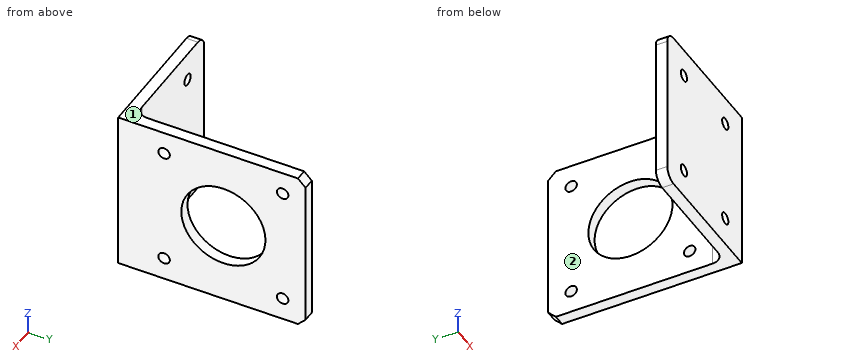
Autodesk Inventor part; units mm, degrees
ref_plane "YZ Plane" through (0, 0, 0) normal (1, 0, 0) x (0, 1, 0)
ref_plane "XZ Plane" through (0, 0, 0) normal (0, 1, 0) x (-1, 0, 0)
ref_plane "XY Plane" through (0, 0, 0) normal (0, 0, 1) x (1, 0, 0)
sketch "Szkic1" plane through (0, 0, 0) normal (0, 0, 1) x (1, 0, 0)
  line L0 (-15.1556, -3.6171) -> (-15.1556, -6.6171)
  line L1 (-15.1556, -6.6171) -> (20.8444, -6.6171)
  line L2 (20.8444, -6.6171) -> (20.8444, 42.3829)
  line L3 (20.8444, 42.3829) -> (17.8444, 42.3829)
  line L4 (17.8444, 42.3829) -> (17.8444, -3.6171)
  line L5 (17.8444, -3.6171) -> (-15.1556, -3.6171)
  point P0 (0, 0)
  dimension "d0" = 3
  dimension "d1" = 36
  dimension "d2" = 49
  dimension "d3" = 3
extrude "Wyciągnięcie proste1" add sketch "Szkic1" along normal blind 43
fillet "Zaokrąglenie1" radius 3 1 edges at (17.8444, -3.6171, 21.5)
sketch "Szkic2" plane through (17.8444, 42.3829, 0) normal (-1, 0, 0) x (0, 0, 1)
  circle A0 centre (21.5033, -21.5) radius 11
  circle A1 centre (21.5, -21.5) radius 16.25
  line L0 (0, 0) -> (0, -43)
  line L1 (0, 0) -> (43, 0)
  line L2 (43, 0) -> (43, -43)
  line L3 (0.5, -0.5) -> (42.5, -0.5)
  line L4 (42.5, -0.5) -> (42.5, -42.5)
  line L5 (42.5, -42.5) -> (0.5, -42.5)
  line L6 (0.5, -42.5) -> (0.5, -0.5)
  point P0 (0, -42.3829)
  point P1 (37, -37)
  point P2 (37, -6)
  point P3 (6, -6)
  point P4 (6, -37)
  dimension "d61" = 42
  dimension "d62" = 42
  dimension "d63" = 0.5
  dimension "d64" = 0.5
  dimension "d65" = 5.5
  dimension "d66" = 5.5
  dimension "d67" = 5.5
  dimension "d68" = 5.5
  dimension "d69" = 5.5
  dimension "d70" = 5.5
  dimension "d71" = 5.5
  dimension "d72" = 5.5
  dimension "d73" = 21
  dimension "d74" = 21
extrude "Wyciągnięcie proste2" cut sketch "Szkic2" against normal blind 43 contours A0
hole "Otwór1" at (17.8444, 5.3829, 6) at (17.8444, 36.3829, 6) at (17.8444, 36.3829, 37) at (17.8444, 5.3829, 37) direction (1, 0, 0) diameter 3 end through all
chamfer "Faza1" distance 2 angle 45 2 edges at (19.3444, 42.3829, 43) (19.3444, 42.3829, 0)
fillet "Zaokrąglenie2" radius 3 2 edges at (-15.1556, -5.1171, 0) (-15.1556, -5.1171, 43)
sketch "Szkic3" plane through (20.8444, -6.6171, 0) normal (0, -1, 0) x (1, 0, 0)
  arc A0 (-33, 43) -> (-36, 40) centre (-33, 40) ccw
  line L0 (-36, 3) -> (-36, 40)
  arc A1 (-36, 3) -> (-33, 0) centre (-33, 3) ccw
  line L1 (-33, 0) -> (0, 0)
  line L2 (0, 0) -> (0, 43)
  line L3 (-33, 43) -> (0, 43)
  point P0 (-20.8444, 0)
  point P1 (-28, 7.5)
  point P2 (-8, 7.5)
  point P3 (-28, 35.5)
  point P4 (-8, 35.5)
  dimension "d32" = 20
  dimension "d33" = 20
  dimension "d34" = 36
  dimension "d35" = 8
  dimension "d36" = 8
  dimension "d37" = 7.5
  dimension "d38" = 7.5
  dimension "d39" = 7.5
  dimension "d40" = 7.5
hole "Otwór2" at (-7.1556, -6.6171, 7.5) at (12.8444, -6.6171, 7.5) at (-7.1556, -6.6171, 35.5) at (12.8444, -6.6171, 35.5) direction (0, 1, 0) diameter 3 end through all
sketch "Szkic4" plane through (14.8444, -3.6171, 43) normal (0, 1, 0) x (1, 0, 0)
  circle A0 centre (-2, 7.5) radius 1.5
  circle A1 centre (-2, 35.5) radius 1.5
  circle A2 centre (-2, 7.5) radius 3.1
  circle A3 centre (-2, 35.5) radius 3.1
  point P0 (-14.8444, 43)
  dimension "d48" = 6.2
  dimension "d49" = 6.2
extrude "Wyciągnięcie proste3" cut sketch "Szkic4" along normal blind 2
properties part number "CNCM_ALU_X_Axis_Nema_17_Mount"
For this review, take the finished solid that the model builds, in its own axes (mm). Face numbers are marked on the shaded views. A direction names the side the tool comes from. Give positions to 0.01 mm unless a question says otherwise; leave off trailing zeros. Order: outer loops, then holes, each group sorted by start corner. A loop starts at its lowest first (then second) coordinate and runs counter-clockwise, first axis right, second up. Notation, with made-up numbers: (65, 70.25) - (107, 70.25) arc R23 ccw to (107, 80.25) - close; hole circle Ø7 at (14, 44.25). An arc over 180 degrees is marked (long way). Answer as a JSON object with one key per item and string values. Group by question number.
Item 1: Take a section at C-C on y = 4.5. Give the boundary of the cut face in (x, z).
Item 2: Take a section at B-B on z = 22. Give the boundary of the cut face in (x, y), and give its area (3 significant figures).
Item 3: Clearance check with flat-ended pins moving along their axes: pin 1 Ø4 at (y, z) = (36.38, 6) entering from -X; pin 2 Ø2.5 at (y, z) = (36.38, 37) entering from -X; pin 3 Ø1.5 at (x, z) = (12.5, 10.5) entering from +Y. State where each tip first meets the part, or that it passes through.
Item 4: Take a section at A-A on y = 19. Give the boundary of the cut face in (x, z).
Item 5: Machinability: for the marked faces 1 and 2, which of the approach directions +Z, -Z, +X, -X, +Y, -Y give a long, thin tool a straight path to every point of the face, cutting with its end or side? Answer none if there is none.
Item 6: Wall thickness on line 1 along Y through (x, z) = (18.85, 37); line 2 along X through (y, z) = (-4, 35); line 3 along X through (y, z) = (4, 10): over which ranges is each line inside the solid? List them lowest first.
Item 7: Take a section at D-D on x = -1.5. Give the boundary of the cut face in (y, z).
Reported:
{
 "1": {"outline": "(17.84, 0) - (20.84, 0) - (20.84, 4.79) - (17.84, 4.79) - close; (17.84, 7.21) - (20.84, 7.21) - (20.84, 35.79) - (17.84, 35.79) - close; (17.84, 38.21) - (20.84, 38.21) - (20.84, 43) - (17.84, 43) - close"},
 "2": {"outline": "(-15.16, -6.62) - (20.84, -6.62) - (20.84, 9.89) - (17.84, 9.89) - (17.84, -0.62) arc R3 cw to (14.84, -3.62) - (-15.16, -3.62) - close; (17.84, 31.87) - (20.84, 31.87) - (20.84, 42.38) - (17.84, 42.38) - close", "area": "182 mm^2"},
 "3": {"pin 1": "x = 17.84", "pin 2": "through", "pin 3": "y = -3.62"},
 "4": {"outline": "(17.84, 0) - (20.84, 0) - (20.84, 10.67) - (17.84, 10.67) - close; (17.84, 32.34) - (20.84, 32.34) - (20.84, 43) - (17.84, 43) - close"},
 "5": {"face 1": "+Z, +X, -X, +Y, -Y", "face 2": "+Z, -Z, -X, +Y"},
 "6": {"line 1": "-6.62 to 3.88, 6.88 to 34.88, 37.88 to 42.38", "line 2": "-15.16 to -8.57, -5.74 to 11.43, 14.26 to 20.84", "line 3": "17.84 to 20.84"},
 "7": {"outline": "(-6.62, 0) - (-3.62, 0) - (-3.62, 43) - (-6.62, 43) - close"}
}
